Design review of the part built by this model. Coordinates are the model's own, in mm. A direction names the side the tool comes from. Give positions to 0.01 mm unless a question says otherwise; leave off trailing zeros. Loops run counter-clockwise (first coordinate to the right, second up) from the corner with the lowest first, then second, coordinate; pieces in that order, holes last. Notation, with made-up numbers: (42.25, 42.5) -> (54.25, 42.5) arc R22 cw to (54.25, 64.5) -> close; hole circle Ø5 at (-33, 38.5). An arc over 180 degrees is marked (long way). Use a Markdown table: item, result. Add a question column.
1. For faces 4 (the cylindrical face through (-111.59, 24.65, -1.34)), 5 (the flat face through (-91.535, 45.232, 0.963)), 6 (the flat face through (-91, 33, -8)), list the 3-axis set-ups (+Z, -Z, +X, -X, +Y, -Y) from which the entire face can be reached by the end or side of a thin tool; tool diameter is ignored.
2. Add section A-A (z = -8.5). State the section outline as (x, y) points, and give its area (3 significant figures).
3. For pin 1 Ø8 at (x, y) = (-75, 5) entering from +Z; pin 2 Ø4 at (x, y) = (-9, 38) entering from +Z; pin 3 Ø1.5 at (y, z) = (9.5, -3.5) entering from -X; pin 4 Ø4 at (x, z) = (-93.5, -7.5) entering from -Y, all flat-tipped, find the tip position at first contact; note any pin that passes through.
4. Add section C-C (y = 38). State the section outline as (x, z) points, and give its area (3 significant figures).
5. Draft analysis for pull direction X (two halves, no side actions). For faces 1 (the cylindrical face through (-85.75, 47.04, 3.07)), 2 (the flat face through (-60, 14, -10)), 3 (the flat face through (-29.968, 45.232, -2.965)), state which applies: pulls with the +X half, pulls with the -X half, needs draft (parallel to the pull), parting line crosses it, or undercut.
6. To check wall thickness, follow line 1 (X direction, y = 7, z = 1.25); line 2 (X direction, y = 32.5, z = -0.5); line 3 (Y direction, x = -99, z = -3.5). State the ranges of each line that lie inside material, in increasing order.
7. Add section B-B (y = 20). Count the separate pieces of the cut face and the enclosed holes in it, and give its area (3 significant figures).
```python
from build123d import *
from build123d.topology import SkipClean

# Parameters (mm, degrees)
BOSS_EXTRUDE2_DEPTH = 50
BOSS_EXTRUDE3_START = -6
BOSS_EXTRUDE3_DEPTH = 6
BOSS_EXTRUDE4_START = 44
BOSS_EXTRUDE4_DEPTH = 44
FILLET1_R           = 5
FILLET2_R           = 3
CUT_EXTRUDE3_DEPTH  = 2.5
SKETCH6_W           = 32
SKETCH6_H           = 8
CUT_EXTRUDE4_DEPTH  = 10


with BuildPart() as part:
    # Sketch1 → Boss-Extrude2 (new body)
    with BuildSketch(Plane(origin=(0, 0, 0), x_dir=(1, 0, 0), z_dir=(0, 1, 0))):
        with BuildLine():
            Line((0, 10), (0, 6.5))
            ThreePointArc((0, 6.5), (4.596194, 4.596194), (6.5, 0))
            ThreePointArc((6.5, 0), (6.464444, -0.678941), (6.358166, -1.350454))
            Line((6.358166, -1.350454), (9.908394, -1.350454))
            ThreePointArc((9.908394, -1.350454), (9.977072, -0.676779), (10, 0))
            ThreePointArc((10, 0), (7.071068, 7.071068), (0, 10))
        make_face()
        with BuildLine():
            ThreePointArc((0, 10), (-4.1833, 9.082951), (-7.599342, 6.5))
            Line((-7.599342, 6.5), (0, 6.5))
            Line((0, 6.5), (0, 10))
        make_face()
        with BuildLine():
            ThreePointArc((-121.5, 10), (-117.3167, 9.082951), (-113.900658, 6.5))
            Line((-113.900658, 6.5), (-7.599342, 6.5))
            ThreePointArc((-7.599342, 6.5), (-4.1833, 9.082951), (0, 10))
            Line((0, 10), (-121.5, 10))
        make_face()
        with BuildLine():
            ThreePointArc((-7.599342, 6.5), (-9.380656, 3.464576), (-10, 0))
            Line((-10, 0), (-6.5, 0))
            ThreePointArc((-6.5, 0), (-4.596194, 4.596194), (0, 6.5))
            Line((0, 6.5), (-7.599342, 6.5))
        make_face()
        with BuildLine():
            Line((-6.5, 0), (-10, 0))
            ThreePointArc((-10, 0), (-9.977072, -0.676779), (-9.908394, -1.350454))
            Line((-9.908394, -1.350454), (-6.358166, -1.350454))
            ThreePointArc((-6.358166, -1.350454), (-6.464444, -0.678941), (-6.5, 0))
        make_face()
        with BuildLine():
            Line((-115, 0), (-111.5, 0))
            ThreePointArc((-111.5, 0), (-112.119344, 3.464576), (-113.900658, 6.5))
            Line((-113.900658, 6.5), (-121.5, 6.5))
            ThreePointArc((-121.5, 6.5), (-116.903806, 4.596194), (-115, 0))
        make_face()
        with BuildLine():
            Line((-121.5, 6.5), (-113.900658, 6.5))
            ThreePointArc((-113.900658, 6.5), (-117.3167, 9.082951), (-121.5, 10))
            ThreePointArc((-121.5, 10), (-129.03341, 6.576301), (-131.408394, -1.350454))
            Line((-131.408394, -1.350454), (-127.858166, -1.350454))
            ThreePointArc((-127.858166, -1.350454), (-126.551136, 4.090969), (-121.5, 6.5))
        make_face()
    extrude(amount=BOSS_EXTRUDE2_DEPTH)

    # Sketch2 → Boss-Extrude3 (add)
    with BuildSketch(Plane(origin=(0, 50, 0), x_dir=(1, 0, 0), z_dir=(0, 1, 0)).offset(BOSS_EXTRUDE3_START)):
        with BuildLine():
            Line((-84.25, -4.5), (-84.25, 6.5))
            Line((-84.25, 6.5), (-95, 6.5))
            Line((-95, 6.5), (-95, 4))
            ThreePointArc((-95, 4), (-92.87868, 3.12132), (-92, 1))
            ThreePointArc((-92, 1), (-92.87868, -1.12132), (-95, -2))
            Line((-95, -2), (-95, -4.5))
            Line((-95, -4.5), (-84.25, -4.5))
        make_face()
        with BuildLine():
            Line((-105.75, -4.5), (-95, -4.5))
            Line((-95, -4.5), (-95, -2))
            ThreePointArc((-95, -2), (-96.732051, -1.44949), (-97.828427, 0))
            Line((-97.828427, 0), (-105.75, 0))
            Line((-105.75, 0), (-105.75, -4.5))
        make_face()
        with BuildLine():
            Line((-95, 4), (-95, 6.5))
            Line((-95, 6.5), (-105.75, 6.5))
            Line((-105.75, 6.5), (-105.75, 0))
            Line((-105.75, 0), (-97.828427, 0))
            ThreePointArc((-97.828427, 0), (-97.44949, 2.732051), (-95, 4))
        make_face()
        with BuildLine():
            Line((-26.5, 6.5), (-37.25, 6.5))
            Line((-37.25, 6.5), (-37.25, -4.5))
            Line((-37.25, -4.5), (-26.5, -4.5))
            Line((-26.5, -4.5), (-26.5, -2))
            ThreePointArc((-26.5, -2), (-29.5, 1), (-26.5, 4))
            Line((-26.5, 4), (-26.5, 6.5))
        make_face()
        with BuildLine():
            Line((-15.75, 6.5), (-26.5, 6.5))
            Line((-26.5, 6.5), (-26.5, 4))
            ThreePointArc((-26.5, 4), (-24.37868, 3.12132), (-23.5, 1))
            ThreePointArc((-23.5, 1), (-23.543204, 0.492694), (-23.671573, 0))
            Line((-23.671573, 0), (-15.75, 0))
            Line((-15.75, 0), (-15.75, 6.5))
        make_face()
        with BuildLine():
            Line((-26.5, -2), (-26.5, -4.5))
            Line((-26.5, -4.5), (-15.75, -4.5))
            Line((-15.75, -4.5), (-15.75, 0))
            Line((-15.75, 0), (-23.671573, 0))
            ThreePointArc((-23.671573, 0), (-24.767949, -1.44949), (-26.5, -2))
        make_face()
        with BuildLine():
            ThreePointArc((-111.5, 0), (-112.119344, 3.464576), (-113.900658, 6.5))
            ThreePointArc((-113.900658, 6.5), (-125.591496, 9.124673), (-131.408394, -1.350454))
            Line((-131.408394, -1.350454), (-127.858166, -1.350454))
            ThreePointArc((-127.858166, -1.350454), (-122.178941, 6.464444), (-115, 0))
            Line((-115, 0), (-111.5, 0))
        make_face()
        with BuildLine():
            ThreePointArc((-111.591606, -1.350454), (-111.522928, -0.676779), (-111.5, 0))
            Line((-111.5, 0), (-115, 0))
            ThreePointArc((-115, 0), (-115.035556, -0.678941), (-115.141834, -1.350454))
            Line((-115.141834, -1.350454), (-111.591606, -1.350454))
        make_face()
    extrude(amount=BOSS_EXTRUDE3_DEPTH)

    # Sketch3 → Boss-Extrude4 (add)
    with SkipClean():  # the faces are left unmerged after this step: merging them gives an invalid solid
        with BuildSketch(Plane.XZ.offset(-44).offset(BOSS_EXTRUDE4_START)):
            with BuildLine():
                Line((-111.591606, 1.350454), (-115.141834, 1.350454))
                ThreePointArc((-115.141834, 1.350454), (-115.035556, 0.678941), (-115, 0))
                Line((-115, 0), (-111.5, 0))
                ThreePointArc((-111.5, 0), (-111.522928, 0.676779), (-111.591606, 1.350454))
            make_face()
        extrude(amount=-BOSS_EXTRUDE4_DEPTH)

    # Fillet1
    fillet1_edges = [part.edges().sort_by_distance(p)[0] for p in [
        (-105.75, 47, 4.5),
        (-105.75, 47, -6.5),
        (-84.25, 47, -6.5),
        (-84.25, 47, 4.5),
        (-15.75, 47, -6.5),
        (-15.75, 47, 4.5),
        (-37.25, 47, 4.5),
        (-37.25, 47, -6.5),
    ]]
    fillet(fillet1_edges, radius=FILLET1_R)

    # Fillet2
    fillet2_edges = [part.edges().sort_by_distance(p)[0] for p in [
        (-7.599342, 25, -6.5),
        (-113.900658, 25, -6.5),
    ]]
    fillet(fillet2_edges, radius=FILLET2_R)

    # Sketch5 → Cut-Extrude3 (cut)
    with SkipClean():  # the faces are left unmerged after this step: merging them gives an invalid solid
        with BuildSketch(Plane.XZ.offset(-44)):
            Polygon((-21.896884, -1), (-24.198442, 2.986415), (-28.801558, 2.986415), (-31.103116, -1), (-28.801558, -4.986415), (-24.198442, -4.986415), align=None)
            Polygon((-90.401179, -1), (-92.70059, 2.982696), (-97.29941, 2.982696), (-99.598821, -1), (-97.29941, -4.982696), (-92.70059, -4.982696), align=None)
        extrude(amount=-CUT_EXTRUDE3_DEPTH, mode=Mode.SUBTRACT)

    # Sketch6 → Cut-Extrude4 (cut)
    with SkipClean():  # the faces are left unmerged after this step: merging them gives an invalid solid
        with BuildSketch(Plane(origin=(0, 0, -10), x_dir=(-1, 0, 0), z_dir=(0, 0, -1))):
            with Locations((91.396524, 21)):
                Rectangle(SKETCH6_W, SKETCH6_H)
            with Locations((91.396524, 29)):
                Rectangle(SKETCH6_W, SKETCH6_H)
            with BuildLine():
                ThreePointArc((68.666891, 25), (60.666891, 33), (52.666891, 25))
                Line((52.666891, 25), (68.666891, 25))
            make_face()
            with BuildLine():
                Line((68.666891, 25), (52.666891, 25))
                ThreePointArc((52.666891, 25), (60.666891, 17), (68.666891, 25))
            make_face()
            with BuildLine():
                ThreePointArc((20.301131, 25), (31.301131, 14), (42.301131, 25))
                Line((42.301131, 25), (20.301131, 25))
            make_face()
            with BuildLine():
                Line((20.301131, 25), (42.301131, 25))
                ThreePointArc((42.301131, 25), (31.301131, 36), (20.301131, 25))
            make_face()
        extrude(amount=-CUT_EXTRUDE4_DEPTH, mode=Mode.SUBTRACT)


solid = part.part
```
Taken from the geometry:
| question | item | result |
|---|---|---|
| 1 | face 4 | +Y, -Y |
| 1 | face 5 | -Y |
| 1 | face 6 | +Z, -Z |
| 2 | outline | (-126.77, 0) -> (5.27, 0) -> (5.27, 50) -> (-126.77, 50) -> close; hole (-107.4, 17) -> (-75.4, 17) -> (-75.4, 33) -> (-107.4, 33) -> close; hole circle Ø16 at (-60.67, 25); hole circle Ø22 at (-31.3, 25) |
| 2 | area | 5,510 mm^2 |
| 3 | pin 1 | stops at z = -6.5 |
| 3 | pin 2 | stops at z = 1.35 |
| 3 | pin 3 | stops at x = -131.11 |
| 3 | pin 4 | stops at y = 0 |
| 4 | outline | (-131.41, 1.35) arc R10 ccw to (-121.5, -10) -> (0, -10) arc R10 ccw to (10, 0) arc R10 ccw to (9.91, 1.35) -> (6.36, 1.35) arc R6.5 cw to (6.5, 0) arc R6.5 cw to (-6.5, 0) arc R6.5 cw to (-6.36, 1.35) -> (-9.91, 1.35) arc R10 ccw to (-10, 0) arc R10 ccw to (-9.63, -2.69) arc R3 cw to (-12.52, -6.5) -> (-108.98, -6.5) arc R3 cw to (-111.87, -2.69) arc R10 ccw to (-111.5, 0) arc R10 ccw to (-111.59, 1.35) -> (-115.14, 1.35) arc R6.5 cw to (-115, 0) arc R6.5 cw (long way) to (-127.86, 1.35) -> close |
| 4 | area | 598 mm^2 |
| 5 | face 1 | undercut |
| 5 | face 2 | needs draft |
| 5 | face 3 | undercut |
| 6 | line 1 | x = -131.42 to -127.88, -115.12 to -111.58, -9.92 to -6.38, 6.38 to 9.92 |
| 6 | line 2 | x = -131.49 to -127.98, -115.02 to -111.51, -9.99 to -6.48, 6.48 to 9.99 |
| 6 | line 3 | y = 44 to 50 |
| 7 | separate pieces | 4 |
| 7 | enclosed holes | 0 |
| 7 | area | 374 mm^2 |
